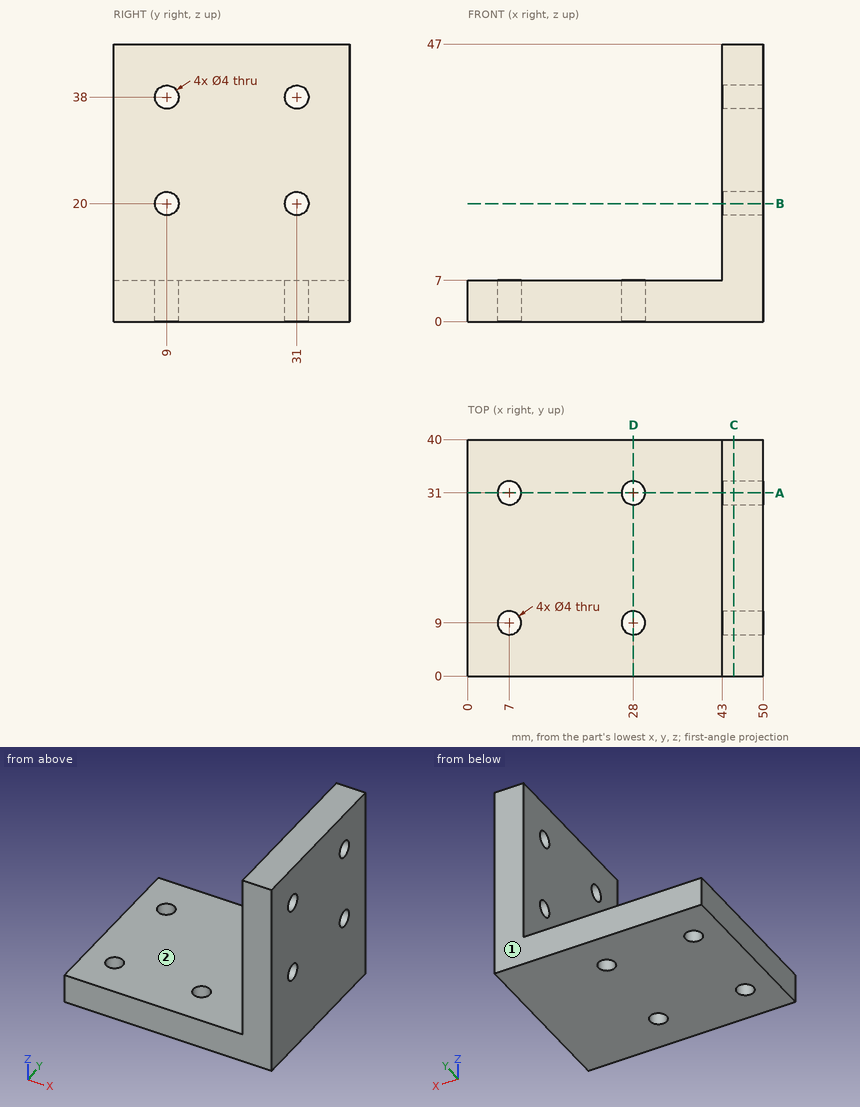
Could you check a few things on this drawing? It's one solid part, dimensions in mm from its lowest x, y, z. A direction names the side the tool comes from. Round coordinates to 2 decimals unless told otherwise and drop trailing zeros. Write each loop counter-clockwise with the first axis right and the second up, starting at its lowest first coordinate (ties: lowest second). Pieces come first, ordered by that corner, then holes. Notation, with made-up numbers: M 22,-17 L 71,-17 A26 cw 71,22 Z; hole C 49.25,56 d3. An arc over 180 degrees is marked long. Answer as CSV lines item,"result". Start each with the question number.
1. I need wall thicknesses on probe 1 along Z at (x, y) = (47.5, 9); probe 2 along Y at (x, z) = (28, 2); probe 3 along X at (y, z) = (21, 35.5). Which ranges of each line are inside material? Lowest first, please.
2. Suppose I cut it at D-D on x = 28. Write out the boundary of the cut face in (y, z).
3. On a 3-axis mill with a long thin cutter (end or side, diameter ignored), from which of +Z, -Z, +X, -X, +Y, -Y can I reach the whole of each face in a straight line? I mean the marked faces 1 and 2. Say none if no direction works.
4. I'm going to push flat-ended pins straight in: pin 1 Ø3 at (x, y) = (7, 31) entering from +Z; pin 2 Ø12 at (y, z) = (21.5, 30) entering from -X; pin 3 Ø4.5 at (y, z) = (31, 38) entering from +X; pin 4 Ø1 at (x, y) = (35.5, 5) entering from +Z. Where does each tip first touch, or does it pass through?
5. Suppose I cut it at C-C on x = 45. Write out the boundary of the cut face in (y, z).
6. Suppose I cut it at A-A on y = 31. Write out the boundary of the cut face in (x, z).
7. Suppose I cut it at B-B on z = 20. Write out the boundary of the cut face in (x, y).
Check result:
1,probe 1,"z = 0 to 18, 22 to 36, 40 to 47"
1,probe 2,"y = 0 to 7, 11 to 29, 33 to 40"
1,probe 3,"x = 43 to 50"
2,outline,"M 0,0 L 7,0 L 7,7 L 0,7 Z; M 11,0 L 29,0 L 29,7 L 11,7 Z; M 33,0 L 40,0 L 40,7 L 33,7 Z"
3,face 1,"+Z, -Z, +X, -X, +Y"
3,face 2,"+Z, -X, +Y, -Y"
4,pin 1,"passes through"
4,pin 2,"stops at x = 43"
4,pin 3,"stops at x = 50"
4,pin 4,"stops at z = 7"
5,outline,"M 0,0 L 40,0 L 40,47 L 0,47 Z; hole C 9,20 d4; hole C 9,38 d4; hole C 31,20 d4; hole C 31,38 d4"
6,outline,"M 0,0 L 5,0 L 5,7 L 0,7 Z; M 9,0 L 26,0 L 26,7 L 9,7 Z; M 30,0 L 50,0 L 50,18 L 43,18 L 43,7 L 30,7 Z; M 43,22 L 50,22 L 50,36 L 43,36 Z; M 43,40 L 50,40 L 50,47 L 43,47 Z"
7,outline,"M 43,0 L 50,0 L 50,7 L 43,7 Z; M 43,11 L 50,11 L 50,29 L 43,29 Z; M 43,33 L 50,33 L 50,40 L 43,40 Z"
